Input: part model. Units: mm. Frame: model coordinates. Face numbers are marked on the shaded views. A direction names the side the tool comes from. Give positions to 0.01 mm unless a question says otherwise; leave off trailing zeros. Order: outer loops, then holes, each group sorted by start corner. A loop starts at its lowest first (then second) coordinate and runs counter-clockwise, first axis right, second up. Notation, with made-up numbers: (-32, -0.5) - (27, -0.5) arc R13 ccw to (27, 15.5) - close; hole circle Ø5 at (38.25, 84.5). An arc over 180 degrees is marked (long way). Answer in a Markdown table with one row per item. Add a question column.
1. Ray query, line 1 (Y direction, x = 0, z = 0.25); line 2 (X direction, y = 0, z = 0.3); line 3 (Y direction, x = -2.5, z = 6.25). Return the intervals inside material, ascending. Write a range as [from, to].
2. Access query for the marked faces 5, 6, 7, 8 and 9. Directions: +Z, -Z, +X, -X, +Y, -Y. A direction counts if a zero-diameter tool reaches every point of the face in a straight line with its end or side. Return the directions, or none.
3. Section query B-B on x = 0. Return loops of the section in (y, z), and give its area (3 significant figures).
4. Section query D-D on x = 4. Return loops of the section in (y, z), and give its area (3 significant figures).
5. Section query A-A on y = 0. Return loops of the section in (x, z), and give its area (3 significant figures).
6. Mould query, pull axis Y, two halves, no side actions, for the marked faces 1, 2, 3 and 4. Classes: released by +Y, released by -Y, zero draft, split by the parting line, or undercut.
7. Contact query for flat-ended pins moving along their axis: pin 1 (4 mm diameter, centred on y = -4, z = 7, fed in from -X); pin 2 (1 mm diameter, centred on y = -12.5, z = 5.5, fed in from -X); pin 3 (11 mm diameter, centred on x = 0, y = 0, fed in from -Z); pin 4 (4 mm diameter, centred on x = -2.5, z = 1.5, fed in from +Y). Output: stop coordinate, or through.
8. Section query C-C on z = 7.25. Count the separate pieces of the cut face and the enclosed holes in it, and give its area (3 significant figures).
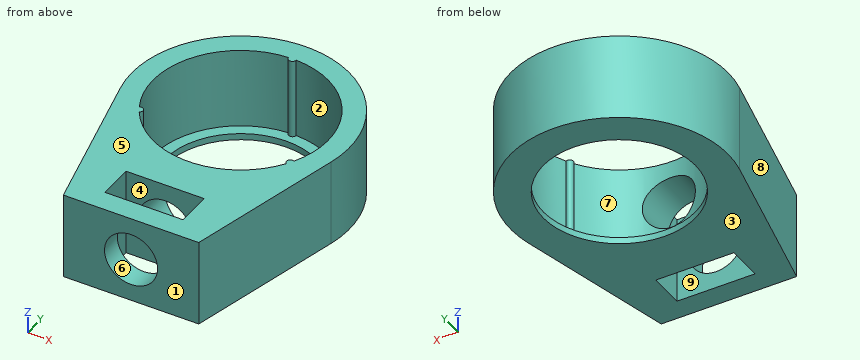
```python
from build123d import *

# Parameters (mm, degrees)
F0_R     = 7
F1_DEPTH = 8
F3_DEPTH = 7.4
F4_R     = 2.45
F5_DEPTH = 12
F6_W     = 7.2
F6_H     = 3.3
F7_DEPTH = 8.001


with BuildPart() as f1:
    # F0 (on Top) → F1 (new body)
    with BuildSketch(Plane.XY):
        with BuildLine():
            Line((6.25, -17), (9.730754, -2.30487))
            ThreePointArc((9.730754, -2.30487), (0, 10), (-9.730754, -2.30487))
            Line((-9.730754, -2.30487), (-6.25, -17))
            Line((-6.25, -17), (6.25, -17))
        make_face()
        Circle(F0_R, mode=Mode.SUBTRACT)
    extrude(amount=F1_DEPTH)

    # F2 (on face) → F3 (cut)
    with BuildSketch(Plane.XY.offset(8)):
        with BuildLine():
            ThreePointArc((0.349917, 8.042391), (0, 7.7), (-0.349917, 8.042391))
            ThreePointArc((-0.349917, 8.042391), (-6.971505, 4.025), (-7.139874, -3.718158))
            ThreePointArc((-7.139874, -3.718158), (-6.668396, -3.85), (-6.789957, -4.324233))
            ThreePointArc((-6.789957, -4.324233), (0, -8.05), (6.789957, -4.324233))
            ThreePointArc((6.789957, -4.324233), (6.668396, -3.85), (7.139874, -3.718158))
            ThreePointArc((7.139874, -3.718158), (6.971505, 4.025), (0.349917, 8.042391))
        make_face()
    extrude(amount=-F3_DEPTH, mode=Mode.SUBTRACT)

    # F4 (on face) → F5 (cut)
    with BuildSketch(Plane.XZ.offset(17)):
        with Locations((0, 4)):
            Circle(F4_R)
    extrude(amount=-F5_DEPTH, mode=Mode.SUBTRACT)

    # F6 (on face) → F7 (cut, through all)
    with BuildSketch(Plane.XY.offset(8)):
        with Locations((0, -13.35)):
            Rectangle(F6_W, F6_H)
    extrude(amount=-F7_DEPTH, mode=Mode.SUBTRACT)


solid = f1.part
```
Answer:
| question | item | result |
|---|---|---|
| 1 | line 1 | y = [-17, -15], [-11.7, -7], [7, 10] |
| 1 | line 2 | x = [-10, -7], [7, 10] |
| 1 | line 3 | y = [-17, -15], [-11.7, -7.65], [7.65, 9.68] |
| 2 | face 5 | +Z, +X, -X, +Y, -Y |
| 2 | face 6 | -Y |
| 2 | face 7 | +Z |
| 2 | face 8 | +Z, -Z, -X, -Y |
| 2 | face 9 | +Z, -Z |
| 3 | outline | (-17, 0) - (-15, 0) - (-15, 1.55) - (-17, 1.55) - close; (-17, 6.45) - (-15, 6.45) - (-15, 8) - (-17, 8) - close; (-11.7, 0) - (-7, 0) - (-7, 0.6) - (-8.05, 0.6) - (-8.05, 1.55) - (-11.7, 1.55) - close; (-11.7, 6.45) - (-8.05, 6.45) - (-8.05, 8) - (-11.7, 8) - close; (7, 0) - (10, 0) - (10, 8) - (7.7, 8) - (7.7, 0.6) - (7, 0.6) - close |
| 3 | area | 37.0 mm² |
| 4 | outline | (-17, 0) - (-5.74, 0) - (-5.74, 0.6) - (-6.99, 0.6) - (-6.99, 8) - (-17, 8) - close; (5.74, 0) - (9.17, 0) - (9.17, 8) - (6.99, 8) - (6.99, 0.6) - (5.74, 0.6) - close |
| 4 | area | 99.0 mm² |
| 5 | outline | (-10, 0) - (-7, 0) - (-7, 0.6) - (-8.05, 0.6) - (-8.05, 8) - (-10, 8) - close; (7, 0) - (10, 0) - (10, 8) - (8.05, 8) - (8.05, 0.6) - (7, 0.6) - close |
| 5 | area | 32.5 mm² |
| 6 | face 1 | released by -Y |
| 6 | face 2 | undercut |
| 6 | face 3 | zero draft |
| 6 | face 4 | undercut |
| 7 | pin 1 | stops at x = -9.8 |
| 7 | pin 2 | stops at x = -7.43 |
| 7 | pin 3 | passes through |
| 7 | pin 4 | stops at y = 9.99 |
| 8 | separate pieces | 1 |
| 8 | enclosed holes | 2 |
| 8 | area | 211 mm² |
